```python
from build123d import *

# Parameters (mm, degrees)
F1_DEPTH = 32
F0_W     = 112
F0_H     = 8.1
F0_H_2   = 3.8
F0_W_2   = 13.5
F0_H_3   = 84
F0_R     = 31.3
F0_W_3   = 40
F0_H_4   = 40
F0_W_4   = 58.5
F0_H_5   = 15.5
F2_DEPTH = 27
F3_DEPTH = 2
F4_DEPTH = 8.1
F5_DEPTH = 10
F6_R     = 3
F7_DEPTH = 14.5
F8_DEPTH = 2


with BuildPart() as f1:
    # F0 (on Top) → F1 (new body)
    with BuildSketch(Plane.XY):
        with BuildLine():
            Line((65, 62), (-65, 62))
            ThreePointArc((-65, 62), (-73.4852813742, 58.4852813742), (-77, 50))
            Line((-77, 50), (-77, -50))
            ThreePointArc((-77, -50), (-73.4852813742, -58.4852813742), (-65, -62))
            Line((-65, -62), (65, -62))
            ThreePointArc((65, -62), (73.4852813742, -58.4852813742), (77, -50))
            Line((77, -50), (77, 50))
            ThreePointArc((77, 50), (73.4852813742, 58.4852813742), (65, 62))
        make_face()
        with BuildLine():
            ThreePointArc((-75, 50), (-72.0710678119, 57.0710678119), (-65, 60))
            Line((-65, 60), (65, 60))
            ThreePointArc((65, 60), (72.0710678119, 57.0710678119), (75, 50))
            Line((75, 50), (75, -50))
            ThreePointArc((75, -50), (72.0710678119, -57.0710678119), (65, -60))
            Line((65, -60), (-65, -60))
            ThreePointArc((-65, -60), (-72.0710678119, -57.0710678119), (-75, -50))
            Line((-75, -50), (-75, 50))
        make_face(mode=Mode.SUBTRACT)
    extrude(amount=F1_DEPTH)

    # F0 (on Top) → F2 (join)
    with BuildSketch(Plane.XY):
        with BuildLine():
            Line((65, 60), (-65, 60))
            ThreePointArc((-65, 60), (-72.0710678119, 57.0710678119), (-75, 50))
            Line((-75, 50), (-75, -50))
            ThreePointArc((-75, -50), (-72.0710678119, -57.0710678119), (-65, -60))
            Line((-65, -60), (65, -60))
            ThreePointArc((65, -60), (72.0710678119, -57.0710678119), (75, -50))
            Line((75, -50), (75, 50))
            ThreePointArc((75, 50), (72.0710678119, 57.0710678119), (65, 60))
        make_face()
        with Locations((-7.5, -44.45)):
            Rectangle(F0_W, F0_H, mode=Mode.SUBTRACT)
        with Locations((-7.5, -33.5)):
            Rectangle(F0_W, F0_H_2, mode=Mode.SUBTRACT)
        with Locations((-7.5, -24.7)):
            Rectangle(F0_W, F0_H_2, mode=Mode.SUBTRACT)
        with Locations((61.75, -12.8)):
            Rectangle(F0_W_2, F0_H_3, mode=Mode.SUBTRACT)
        with Locations((-35, 20)):
            Circle(F0_R, mode=Mode.SUBTRACT)
        with Locations((26.025, 5.8)):
            Rectangle(F0_W_3, F0_H_4, mode=Mode.SUBTRACT)
        with Locations((35.65, 42.15)):
            Rectangle(F0_W_4, F0_H_5, mode=Mode.SUBTRACT)
    extrude(amount=F2_DEPTH)

    # F0 (on Top) → F3 (join)
    with BuildSketch(Plane.XY):
        with Locations((-35, 20)):
            Circle(F0_R)
    extrude(amount=F3_DEPTH)

    # F0 (on Top) → F4 (join)
    with BuildSketch(Plane.XY):
        with Locations((35.65, 42.15)):
            Rectangle(F0_W_4, F0_H_5)
    extrude(amount=F4_DEPTH)

    # F0 (on Top) → F5 (join)
    with BuildSketch(Plane.XY):
        with Locations((61.75, -12.8)):
            Rectangle(F0_W_2, F0_H_3)
    extrude(amount=F5_DEPTH)

    # F6
    f6_edges = [f1.edges().sort_by_distance(p)[0] for p in [
        (55, -12.8, 10),
        (61.75, -54.8, 10),
        (68.5, -12.8, 10),
        (61.75, 29.2, 10),
    ]]
    fillet(f6_edges, radius=F6_R)

    # F0 (on Top) → F7 (join)
    with BuildSketch(Plane.XY):
        with Locations((-7.5, -44.45)):
            Rectangle(F0_W, F0_H)
        with Locations((-7.5, -33.5)):
            Rectangle(F0_W, F0_H_2)
        with Locations((-7.5, -24.7)):
            Rectangle(F0_W, F0_H_2)
    extrude(amount=F7_DEPTH)

    # F0 (on Top) → F8 (join)
    with BuildSketch(Plane.XY):
        with Locations((26.025, 5.8)):
            Rectangle(F0_W_3, F0_H_4)
    extrude(amount=F8_DEPTH)


solid = f1.part
```
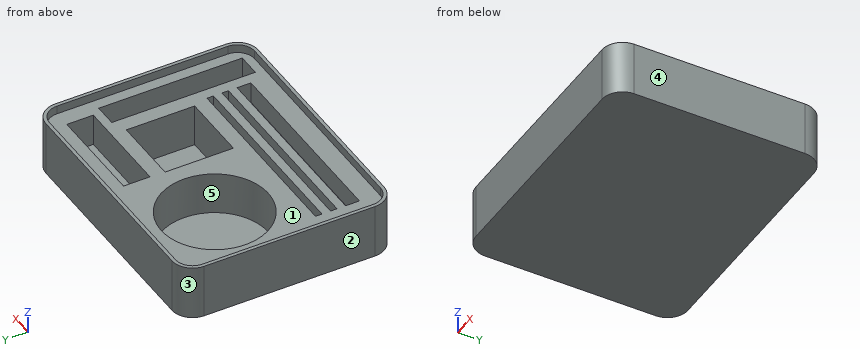
CAD build for the part. Positions are in the model's coordinates, mm. Face numbers are marked on the shaded views. A direction names the side the tool comes from. Coordinates: 2 decimals unless noted, no trailing zeros. Write each loop counter-clockwise with the first axis right and the second up, starting at its lowest first coordinate (ties: lowest second). Pieces come first, ordered by that corner, then holes. Notation, with made-up numbers: (38, 74.5) -> (59, 74.5) arc R28 ccw to (59, 101.5) -> close; hole circle Ø7 at (-22.75, 33). An arc over 180 degrees is marked (long way). Use CSV: the item, a comma, the result in double quotes. Start each with the question number.
Item 1: Drop flat-ended pins along their axis: P1, Ø1.9, axis at x = -29.5, y = -24.5, coming from the +Z side; P2, Ø10, axis at x = -1.5, y = 23.5, coming from the +Z side. Give the stop position or say it passes through.
Item 2: Wall check: probe 1 along Y at (x, z) = (58, 21); probe 2 along Y at (x, z) = (17, 10); probe 3 along Y at (x, z) = (-35, 19). Give the ranges that are in metal, low to high.
Item 3: Two-plate mould, pull along Y, no slides. Class the marked faces 1, 2 and 3: +Y half, -Y half, draft (parallel to the pull), parting line (faces both ways), or undercut.
Item 4: Band-saw the part on A-A, the plane z = 29.5. Write the cut outline in (x, y).
Item 5: Band-saw the part on B-B, the plane y = 20. Write the cut outline in (x, z) (3 decimals), plus the area to 3 significant figures.
Item 6: Band-saw the part on D-D, the plane z = 18. Give the number of separate pieces and of enclosed holes in the cut face, plus the area to 3 significant figures.
Item 7: Tool access for the marked faces 4 and 5: list every direction of +Z, -Z, +X, -X, +Y, -Y with a clear straight run to the whole face (end or side of a thin tool).
Item 8: Band-saw the part on C-C, the plane x = -35. Write the cut outline in (y, z).
Response values:
1,P1,"stops at z = 14.5"
1,P2,"stops at z = 27"
2,probe 1,"y = -62 to -54.8, 29.2 to 34.4, 49.9 to 62"
2,probe 2,"y = -62 to -14.2, 25.8 to 34.4, 49.9 to 62"
2,probe 3,"y = -62 to -48.5, -40.4 to -35.4, -31.6 to -26.6, -22.8 to -11.3, 51.3 to 62"
3,face 1,"undercut"
3,face 2,"draft"
3,face 3,"+Y half"
4,outline,"(-77, -50) arc R12 ccw to (-65, -62) -> (65, -62) arc R12 ccw to (77, -50) -> (77, 50) arc R12 ccw to (65, 62) -> (-65, 62) arc R12 ccw to (-77, 50) -> close; hole (-75, -50) arc R10 ccw to (-65, -60) -> (65, -60) arc R10 ccw to (75, -50) -> (75, 50) arc R10 ccw to (65, 60) -> (-65, 60) arc R10 ccw to (-75, 50) -> close"
5,outline,"(-77, 0) -> (77, 0) -> (77, 32) -> (75, 32) -> (75, 27) -> (68.5, 27) -> (68.5, 13) arc R3 cw to (65.5, 10) -> (58, 10) arc R3 cw to (55, 13) -> (55, 27) -> (46.025, 27) -> (46.025, 2) -> (6.025, 2) -> (6.025, 27) -> (-3.7, 27) -> (-3.7, 2) -> (-66.3, 2) -> (-66.3, 27) -> (-75, 27) -> (-75, 32) -> (-77, 32) -> close"
5,area,"1,390 mm2"
6,separate pieces,"1"
6,enclosed holes,"7"
6,area,"10,500 mm2"
7,face 4,"+Z, -Z, +X, +Y, -Y"
7,face 5,"+Z"
8,outline,"(-62, 0) -> (62, 0) -> (62, 32) -> (60, 32) -> (60, 27) -> (51.3, 27) -> (51.3, 2) -> (-11.3, 2) -> (-11.3, 27) -> (-22.8, 27) -> (-22.8, 14.5) -> (-26.6, 14.5) -> (-26.6, 27) -> (-31.6, 27) -> (-31.6, 14.5) -> (-35.4, 14.5) -> (-35.4, 27) -> (-40.4, 27) -> (-40.4, 14.5) -> (-48.5, 14.5) -> (-48.5, 27) -> (-60, 27) -> (-60, 32) -> (-62, 32) -> close"
